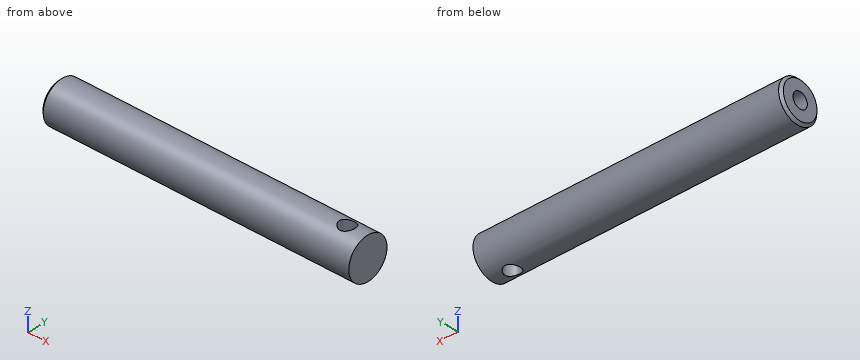
```python
from build123d import *

# Parameters (mm, degrees)
SKETCH1_R               = 6.35
BASE_EXTRUDE_DEPTH      = 95.25
SKETCH2_R               = 2.38125
CUT_EXTRUDE1_DEPTH      = 7.35
CUT_EXTRUDE1_DEPTH_BACK = 7.35
SKETCH3_R               = 2.38125
CUT_EXTRUDE2_DEPTH      = 25.4
CHAMFER2_SIZE           = 0.762


with BuildPart() as part:
    # Sketch1 → Base-Extrude (new body)
    with BuildSketch(Plane(origin=(0, 0, 0), x_dir=(0, 0, -1), z_dir=(1, 0, 0))):
        Circle(SKETCH1_R)
    extrude(amount=BASE_EXTRUDE_DEPTH)

    # Sketch2 → Cut-Extrude1 (cut, two sides)
    with BuildSketch(Plane.XY) as cut_extrude1_sk:
        with Locations((88.9, 0)):
            Circle(SKETCH2_R)
    extrude(amount=CUT_EXTRUDE1_DEPTH, mode=Mode.SUBTRACT)
    extrude(cut_extrude1_sk.sketch, amount=-CUT_EXTRUDE1_DEPTH_BACK, mode=Mode.SUBTRACT)

    # Sketch3 → Cut-Extrude2 (cut)
    with BuildSketch(Plane.ZY):
        Circle(SKETCH3_R)
    extrude(amount=-CUT_EXTRUDE2_DEPTH, mode=Mode.SUBTRACT)

    # Chamfer2
    chamfer2_edges = [part.edges().sort_by_distance(p)[0] for p in [
        (0, 0, 6.35),
    ]]
    chamfer(chamfer2_edges, length=CHAMFER2_SIZE)


solid = part.part
```
For this review, take the finished solid that the model builds, in its own axes (mm). Round coordinates to 2 decimals unless told otherwise and drop trailing zeros. Write each loop counter-clockwise with the first axis right and the second up, starting at its lowest first coordinate (ties: lowest second). Pieces come first, ordered by that corner, then holes. Notation, with made-up numbers: (0, 12.5) -> (29, 12.5) arc R16 ccw to (29, 29.5) -> close; hole circle Ø6 at (-4.5, -38). An arc over 180 degrees is marked (long way). One line per question, with ' | ' between items. Start each with the question number.
1) Add section B-B (y = 0). Write out the cut boundary in (x, z).
2) Wall thickness on line 1 along Y through (x, z) = (19, 0); line 2 along X through (y, z) = (0, -1.5); line 3 along Y through (x, z) = (90, -3.75): over which ranges is each line inside the solid? List them lowest first.
3) Add section A-A (z = 0). Write out the cut boundary in (x, y), and give its area (3 significant figures).
4) Add section D-D (x = 47.5). Write out the cut boundary in (y, z).
5) Add section C-C (x = 9). Write out the cut boundary in (y, z).
6) For pin 1 Ø2 at (x, y) = (29, -4) entering from +Z; pin 2 Ø2 at (x, z) = (19.5, -2.5) entering from +Y; pin 3 Ø1 at (x, z) = (23.5, -2.5) entering from -Y; pin 4 Ø4.5 at (x, y) = (88.9, 0) entering from -Z, all flat-tipped, find the tip position at first contact; note any pin that passes through.
Reported:
1) outline: (0, -5.59) -> (0.76, -6.35) -> (86.52, -6.35) -> (86.52, 6.35) -> (0.76, 6.35) -> (0, 5.59) -> (0, 2.38) -> (25.4, 2.38) -> (25.4, -2.38) -> (0, -2.38) -> close; (91.28, -6.35) -> (95.25, -6.35) -> (95.25, 6.35) -> (91.28, 6.35) -> close
2) line 1: y = -6.35 to -2.38, 2.38 to 6.35 | line 2: x = 25.4 to 86.52, 91.28 to 95.25 | line 3: y = -5.12 to -2.11, 2.11 to 5.12
3) outline: (0, -5.59) -> (0.76, -6.35) -> (95.25, -6.35) -> (95.25, 6.35) -> (0.76, 6.35) -> (0, 5.59) -> (0, 2.38) -> (25.4, 2.38) -> (25.4, -2.38) -> (0, -2.38) -> close; hole circle Ø4.76 at (88.9, 0) | area: 1,070 mm²
4) outline: circle Ø12.7 at (0, 0)
5) outline: circle Ø12.7 at (0, 0); hole circle Ø4.76 at (0, 0)
6) pin 1: stops at z = 5.6 | pin 2: stops at y = 6.17 | pin 3: stops at y = -6.03 | pin 4: passes through
